CAD build for the part. Positions are in the model's coordinates, mm. Face numbers are marked on the shaded views. A direction names the side the tool comes from. Round coordinates to 2 decimals unless told otherwise and drop trailing zeros. Loops run counter-clockwise (first coordinate to the right, second up) from the corner with the lowest first, then second, coordinate; pieces in that order, holes last. Notation, with made-up numbers: M 33.5,-19.75 L 77.5,-19.75 A17 ccw 77.5,13.25 Z; hole C 2.5,-39.5 d8. An arc over 180 degrees is marked long. Use one line per item in the form item = value.
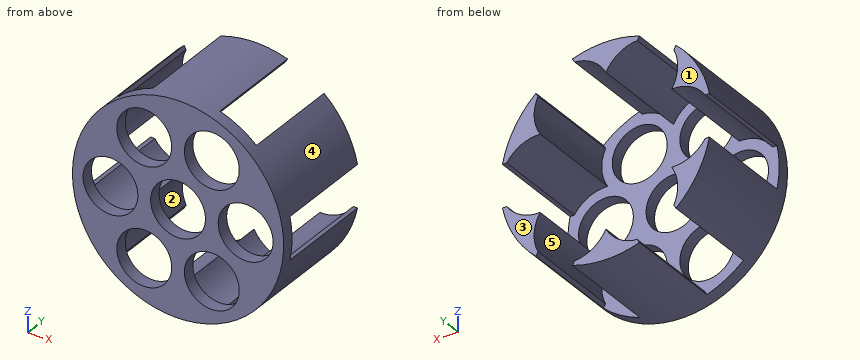
Autodesk Inventor part; units mm, degrees
ref_plane "YZ Plane" through (0, 0, 0) normal (1, 0, 0) x (0, 1, 0)
ref_plane "XZ Plane" through (0, 0, 0) normal (0, 1, 0) x (-1, 0, 0)
ref_plane "XY Plane" through (0, 0, 0) normal (0, 0, 1) x (1, 0, 0)
sketch "스케치1" plane through (0, 0, 0) normal (0, 1, 0) x (-1, 0, 0)
  circle A0 centre (0, 0) radius 25
  circle A1 centre (16, 0) radius 6.5
  circle A2 centre (8, 13.8564) radius 6.5
  circle A3 centre (-8, 13.8564) radius 6.5
  circle A4 centre (-16, 0) radius 6.5
  circle A5 centre (-8, -13.8564) radius 6.5
  circle A6 centre (8, -13.8564) radius 6.5
  circle A7 centre (0, 0) radius 6.5
  dimension "d0" = 50
  dimension "d1" = 13
  dimension "d2" = 16
  dimension "d5" = 360
  dimension "d7" = 13
extrude "돌출1" add sketch "스케치1" along normal blind 3
sketch "스케치2" plane through (0, 3, 0) normal (0, 1, 0) x (1, 0, 0)
  circle A0 centre (-16, 0) radius 6.5
  circle A1 centre (-8, 13.8564) radius 6.5
  circle A2 centre (8, 13.8564) radius 6.5
  circle A3 centre (8, -13.8564) radius 6.5
  circle A4 centre (-8, -13.8564) radius 6.5
  circle A5 centre (0, 0) radius 25
  arc A6 (-15.5707, 8.9898) -> (-15.5707, -8.9898) centre (-16, 0) ccw
  arc A7 (0, 17.9795) -> (-15.5707, 8.9898) centre (-8, 13.8564) ccw
  arc A8 (15.5707, 8.9898) -> (0, 17.9795) centre (8, 13.8564) ccw
  arc A9 (15.5707, -8.9898) -> (15.5707, 8.9898) centre (16, 0) ccw
  arc A10 (0, -17.9795) -> (15.5707, -8.9898) centre (8, -13.8564) ccw
  arc A11 (-15.5707, -8.9898) -> (0, -17.9795) centre (-8, -13.8564) ccw
  line L0 (25, -5) -> (-25, -5)
  line L1 (-25, -5) -> (-25, 5)
  line L2 (-25, 5) -> (25, 5)
  line L3 (25, 5) -> (25, -5)
  line L4 (25, -5) -> (-25, 5) construction
  line L5 (-25, -5) -> (25, 5) construction
  line L6 (-8.1699, -24.1506) -> (-16.8301, -19.1506)
  line L7 (-16.8301, -19.1506) -> (8.1699, 24.1506)
  line L8 (16.8301, 19.1506) -> (-8.1699, -24.1506)
  line L9 (8.1699, 24.1506) -> (16.8301, 19.1506)
  line L10 (16.8301, -19.1506) -> (8.1699, -24.1506)
  line L11 (8.1699, -24.1506) -> (-16.8301, 19.1506)
  line L12 (-8.1699, 24.1506) -> (16.8301, -19.1506)
  line L13 (-16.8301, 19.1506) -> (-8.1699, 24.1506)
  line L14 (25, 5) -> (25, -5)
  line L15 (25, -5) -> (-25, -5)
  line L16 (-25, 5) -> (25, 5)
  line L17 (-25, -5) -> (-25, 5)
  line L18 (8.1699, 24.1506) -> (16.8301, 19.1506)
  line L19 (16.8301, 19.1506) -> (-8.1699, -24.1506)
  line L20 (-16.8301, -19.1506) -> (8.1699, 24.1506)
  line L21 (-8.1699, -24.1506) -> (-16.8301, -19.1506)
  line L22 (-16.8301, 19.1506) -> (-8.1699, 24.1506)
  line L23 (-8.1699, 24.1506) -> (16.8301, -19.1506)
  line L24 (8.1699, -24.1506) -> (-16.8301, 19.1506)
  line L25 (16.8301, -19.1506) -> (8.1699, -24.1506)
  point P0 (16, 0)
  dimension "d17" = 50
  dimension "d18" = 10
  dimension "d21" = 360
extrude "돌출2" add sketch "스케치2" along normal blind 24 contours L2 A5 L11 A7 A6 | A6 A5 L2 | L0 A5 A6 | A6 A11 L7 A5 L0 | L11 A5 A7 | A11 A5 L7 | A5 L12 A7 | L2 A5 A9 | A9 A8 L8 A5 L2 | L12 A5 L7 A8 A7 | A11 L8 A5 | L0 A5 L12 A10 A9 | A9 A5 L0 | A11 A10 L11 A5 L8 | L7 A5 A8 | A10 A5 L11 | A8 A5 L8 | L12 A5 A10
extrude "돌출3" cut sketch "스케치2" along normal blind 27 contours A0 L0 L2 | A0 L2 L11 L7 L0 | A0 L0 A6 L2 | L11 A1 L12 L7 L2 | L2 L7 L11 | L7 L11 L0 | L0 L11 L8 A4 L7 | A6 A5 L2 | L7 L12 L2 | L2 L12 L8 L0 L11 L7 | L11 A1 L12 | L0 A5 A6 | L0 L8 L11 | A4 L8 L7 | L1 L2 A5 | A5 L0 L1 | L12 L7 A2 L8 L2 | L2 L8 L12 | L11 A7 L12 A1 | L8 L12 L0 | L0 L12 A3 L11 L8 | A4 L8 A11 L7 | L11 A5 A7 | L11 L13 A5 | L2 A9 L0 L12 L8 | L7 A2 L8 | A11 A5 L7 | A5 L6 L7 | A3 L12 L11 | L13 L12 A5 | A5 L12 A7 | L2 A5 A9 | L7 A8 L8 A2 | A11 L8 A5 | A5 L8 L6 | A9 A5 L0 | A3 L12 A10 L11 | L3 L0 A5 | A5 L2 L3 | L7 A5 A8 | A10 A5 L11 | L7 L9 A5 | A8 A5 L8 | A5 L9 L8 | A5 L10 L11 | L12 A5 A10 | L12 L10 A5
properties part number "hand_joy_cover"
1. Cut at D-D on x = -2.5. Write the cut outline in (y, z), and give its area (3 significant figures).
Completed:
outline = M 0,-24.87 L 27,-24.87 L 27,-20.98 L 3,-20.98 L 3,-17.32 L 0,-17.32 Z; M 0,-10.39 L 3,-10.39 L 3,-6 L 0,-6 Z; M 0,6 L 3,6 L 3,10.39 L 0,10.39 Z; M 0,17.32 L 3,17.32 L 3,20.98 L 27,20.98 L 27,24.87 L 0,24.87 Z
area = 259 mm2
2. Drop flat-ended pins along their axis: P1, Ø21, axis at x = 0, z = 0, coming from the +Y side; P2, Ø1.5, axis at y = 8, z = 16.5, coming from the +X side; P3, Ø10, axis at x = -14.5, y = 9, coming from the +Z side. Give the stop position or say it passes through.
Completed:
P1 = 3
P2 = 19.41
P3 = 18.71
3. Cut at B-B on y = 25. State how many separate pieces and enclosed holes the cut face has, and give its area (3 significant figures).
Completed:
separate_pieces = 6
enclosed_holes = 0
area = 295 mm2
4. Cut at C-C on x = 21. Write the cut outline in (y, z).
Completed:
outline = M 0,-13.56 L 27,-13.56 L 27,-7.48 L 3,-7.48 L 3,-4.15 L 0,-4.15 Z; M 0,4.15 L 3,4.15 L 3,7.48 L 27,7.48 L 27,13.56 L 0,13.56 Z
5. Tool access for the marked faces 1 and 2: list every direction of +Z, -Z, +X, -X, +Y, -Y with a clear straight run to the whole face (end or side of a thin tool).
Completed:
face_1 = +Z, -Z, +X, -X, +Y
face_2 = +Y
6. Pull direction X, two halves, no side cores. Call the marked faces 3, 4 and 5: +X half, -X half, draft (parallel to the pull), parting line (faces both ways), or undercut.
Completed:
face_3 = draft
face_4 = parting line
face_5 = undercut
7. Probe line 1 along Z through (x, y) = (-8, 1.7); line 2 along X through (y, z) = (1.75, 14.5); line 3 along Y through (x, z) = (8, 22.5). List the from-to ranges inside material, lowest first. Write a range as from..to.
Completed:
line_1 = -23.69..-20.36, -7.36..7.36, 20.36..23.69
line_2 = -20.37..-14.47, -1.53..1.53, 14.47..20.37
line_3 = 0..3
8. Cut at A-A on z = 0. Write the cut outline in (x, y), and give its area (3 significant figures).
Completed:
outline = M -25,0 L -22.5,0 L -22.5,3 L -25,3 Z; M -9.5,0 L -6.5,0 L -6.5,3 L -9.5,3 Z; M 6.5,0 L 9.5,0 L 9.5,3 L 6.5,3 Z; M 22.5,0 L 25,0 L 25,3 L 22.5,3 Z
area = 33.0 mm2
